Part model, mm, in its own coordinate system. Face numbers are marked on the shaded views. Give positions to 0.01 mm unless a question says otherwise; leave off trailing zeros. Order: outer loops, then holes, each group sorted by start corner. A loop starts at its lowest first (then second) coordinate and runs counter-clockwise, first axis right, second up.
Autodesk Inventor part; units mm, degrees
ref_plane "YZ Plane" through (0, 0, 0) normal (1, 0, 0) x (0, 1, 0)
ref_plane "XZ Plane" through (0, 0, 0) normal (0, 1, 0) x (-1, 0, 0)
ref_plane "XY Plane" through (0, 0, 0) normal (0, 0, 1) x (1, 0, 0)
sketch "Sketch1" plane through (0, 0, 0) normal (0, 1, 0) x (-1, 0, 0)
  circle A0 centre (0, 0) radius 5
  circle A1 centre (0, 0) radius 1.6
  dimension "d0" = 10
  dimension "d1" = 3.2
extrude "Extrusion1" add sketch "Sketch1" along normal blind 45
sketch "Sketch2" plane through (0, 45, 0) normal (0, 1, 0) x (1, 0, 0)
  circle A0 centre (0, 3) radius 0.75
  circle A1 centre (0, -3) radius 0.75
  point P0 (0, 0)
  dimension "d4" = 1.5
  dimension "d5" = 1.5
  dimension "d6" = 6
  dimension "d7" = 3
  dimension "d8" = 0
  dimension "d10" = 0
extrude "Extrusion2" cut sketch "Sketch2" against normal through all
sketch "Sketch3" plane through (0, 0, 0) normal (0, -1, 0) x (1, 0, 0)
  circle A0 centre (0, 0) radius 4.5
  dimension "d13" = 9
extrude "Extrusion3" cut sketch "Sketch3" against normal blind 35
sketch "Sketch4" plane through (0, 0, 0) normal (1, 0, 0) x (0, 1, 0)
  line L0 (0, -5) -> (0, 5)
  line L1 (0, 5) -> (5.7735, -5)
  line L2 (0, -5) -> (45, -5)
  line L3 (0, 5) -> (11.547, 5) construction
  line L4 (5.7735, -5) -> (0, -5)
  line L5 (0, 5) -> (0, -5)
  point P0 (0, 0)
  dimension "d16" = 60
extrude "Extrusion4" cut sketch "Sketch4" along normal through all both and the other way through all
sketch "Sketch5" plane through (0, 45, 0) normal (0, 1, 0) x (1, 0, 0)
  circle A0 centre (0, 0) radius 5
  circle A1 centre (0, 0) radius 4
  dimension "d19" = 10
  dimension "d20" = 8
extrude "Extrusion5" cut sketch "Sketch5" against normal blind 5
properties part number "End-tip Coupler" material "Copper"
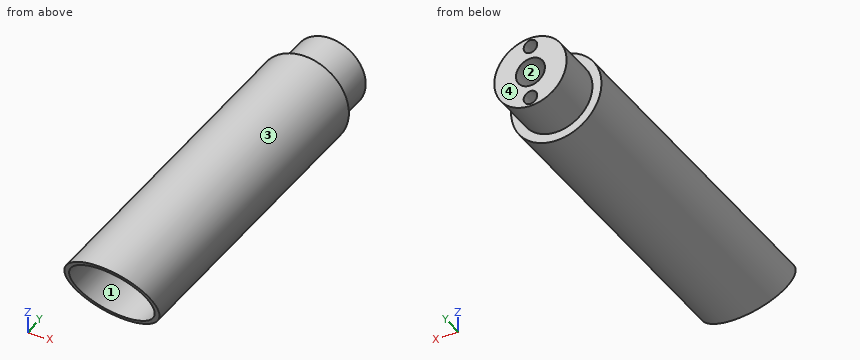
Item 1: Pull direction Z, two halves, no side cores. Call the marked faces 1, 2, 3 and 4: released by +Z, released by -Z, zero draft, split by the parting line, or undercut.
Item 2: Drill centre lines: probe 1 along Z at (x, y) = (0, 39.75); probe 2 along X at (y, z) = (38.5, 3); probe 3 along Z at (x, y) = (0, 41). Where is each one in solid material? Low to high.
Item 3: Band-saw the part on B-B on x = 0. List the corners of the cut face in (y, z), plus the area to 3 significant figures.
Item 4: Band-saw the part on A-A on z = -3. List the corners of the cut face in (x, y), plus the area to 3 significant figures.
Item 5: Band-saw the part on C-C on y = 20.5. List the corners of the cut face in (x, z).
Item 6: Drop flat-ended pins along their axis: P1, Ø1.2, axis at x = 0, z = -3, coming from the +Y side; P2, Ø6, axis at x = 0.5, z = 0.5, coming from the -Y side; P3, Ø5, axis at y = 31.5, z = 2.5, coming from the +X side; P4, Ø4.5, axis at x = -2, z = 2, coming from the -Y side. Give the stop position or say it passes through.
Item 7: Band-saw the part on D-D on x = 3. List the corners of the cut face in (y, z), plus the area to 3 significant figures.
Working result:
1. face 1: undercut
1. face 2: undercut
1. face 3: split by the parting line
1. face 4: zero draft
2. probe 1: z = -5 to -3.75, -2.25 to -1.6, 1.6 to 2.25, 3.75 to 5
2. probe 2: x = -4 to -0.75, 0.75 to 4
2. probe 3: z = -4 to -3.75, -2.25 to -1.6, 1.6 to 2.25, 3.75 to 4
3. outline: (0, 5) - (0.29, 4.5) - (35, 4.5) - (35, 3.75) - (45, 3.75) - (45, 4) - (40, 4) - (40, 5) - close; (5.48, -4.5) - (5.77, -5) - (40, -5) - (40, -4) - (45, -4) - (45, -3.75) - (35, -3.75) - (35, -4.5) - close; (35, -2.25) - (45, -2.25) - (45, -1.6) - (35, -1.6) - close; (35, 1.6) - (45, 1.6) - (45, 2.25) - (35, 2.25) - close
3. area: 60.1 mm2
4. outline: (-4, 4.62) - (-3.35, 4.62) - (-3.35, 35) - (-0.75, 35) - (-0.75, 45) - (-2.65, 45) - (-2.65, 40) - (-4, 40) - close; (0.75, 35) - (3.35, 35) - (3.35, 4.62) - (4, 4.62) - (4, 40) - (2.65, 40) - (2.65, 45) - (0.75, 45) - close
4. area: 90.7 mm2
5. outline: circle Ø10 at (0, 0); hole circle Ø9 at (0, 0)
6. P1: passes through
6. P2: stops at y = 35
6. P3: stops at x = 5
6. P4: stops at y = 0.43
7. outline: (0.58, 4) - (0.95, 3.35) - (35, 3.35) - (35, -3.35) - (4.82, -3.35) - (5.2, -4) - (40, -4) - (40, -2.65) - (45, -2.65) - (45, 2.65) - (40, 2.65) - (40, 4) - close
7. area: 108 mm2
